Build history of the part. All positions in model axes, mm. A direction names the side the tool comes from. Round coordinates to 2 decimals unless told otherwise and drop trailing zeros. Write each loop counter-clockwise with the first axis right and the second up, starting at its lowest first coordinate (ties: lowest second). Pieces come first, ordered by that corner, then holes.
1) Saw through at B-B (z = 2). Write the cut outline in (x, y).
2) Saw through at C-C (x = 40). Write the cut outline in (y, z).
3) Saw through at A-A (y = 3.8). State how many separate pieces and enclosed holes the cut face has, plus the area to 3 significant figures.
4) Pull direction Z, two halves, no side cores. Call faces 1 (the cylindrical face through (-79.14, 1.01, 17.1)), 2 (the flat face through (-1, 3, -14)), 3 (the cylindrical face through (-79.14, 1.01, -17.1)): +Z half, -Z half, draft (parallel to the pull), parting line (faces both ways), or undercut.
5) Flat gauge pins, fed straight in: pin 1 (2.5 mm diameter, centred on y = 4, z = 2.5, fed in from +X); pin 2 (12 mm diameter, centred on x = 12, z = -5.5, fed in from +Y); pin 3 (2.5 mm diameter, centred on x = -25, y = 3.5, fed in from -Z); pin 4 (2.5 mm diameter, centred on x = 75, z = 13, fed in from -Y). Where does each tip first touch, or does it go through?
6) Saw through at D-D (x = 70). Write the cut outline in (y, z).
7) Wall check: probe 1 along Z at (x, y) = (75, 1.8); probe 2 along X at (y, z) = (1.85, 13); probe 3 along Z at (x, y) = (14, 3.05). Give the ranges that are in metal, low to high.
8) Which spindle directions (+Z, -Z, +X, -X, +Y, -Y) get a long thin tool onto all of the face, cutting with end or side? Do faces 4 (the flat face through (-1, 2, 0)), 5 (the flat face through (-1, 3, -16)), 6 (the flat face through (78, 3, 0)), 7 (the flat face through (-76, 3, 0)). Say none if no direction does.
from build123d import *

# Parameters (mm, degrees)
SKETCH1_W                    = 160
SKETCH1_H                    = 36
BOSS_EXTRUDE1_DEPTH          = 2
SKETCH2_W                    = 130
SKETCH2_H                    = 2
SKETCH2_W_2                  = 2
SKETCH2_H_2                  = 16
BOSS_EXTRUDE2_DEPTH          = 3
CSK_FOR_M3_SFHCS1_AT_2_COUNT = 2
CSK_FOR_M3_SFHCS1_AT_2_PITCH = 26
CIRPATTERN1_COUNT            = 2
FILLET1_R                    = 3
FILLET2_R                    = 1


with BuildPart() as part:
    # Sketch1 → Boss-Extrude1 (new body)
    with BuildSketch(Plane(origin=(0, 0, 0), x_dir=(1, 0, 0), z_dir=(0, 1, 0))):
        Rectangle(SKETCH1_W, SKETCH1_H)
    extrude(amount=BOSS_EXTRUDE1_DEPTH)

    # Sketch2 → Boss-Extrude2 (add)
    with BuildSketch(Plane(origin=(0, 2, 0), x_dir=(1, 0, 0), z_dir=(0, 1, 0))):
        with Locations((0, 15)):
            Rectangle(SKETCH2_W, SKETCH2_H)
        with Locations((77, 0)):
            Rectangle(SKETCH2_W_2, SKETCH2_H_2)
    boss_extrude2 = extrude(amount=BOSS_EXTRUDE2_DEPTH)

    # Sketch7 → CSK for M3 SFHCS1 (revolve, cut)
    with BuildSketch(Plane(origin=(75, 0, -13), x_dir=(0, 0, -1), z_dir=(1, 0, 0))):
        Polygon((0, 0), (0, 11.021463052), (1.7, 10), (1.7, 1.66), (3.36, 0), align=None)
    csk_for_m3_sfhcs1 = revolve(axis=Axis((75, -6.35, -13), (0, 1, 0)), mode=Mode.SUBTRACT)

    # CSK for M3 SFHCS1 at 2: CSK for M3 SFHCS1 ×2
    with Locations(*[(0, 0, i * CSK_FOR_M3_SFHCS1_AT_2_PITCH) for i in range(1, CSK_FOR_M3_SFHCS1_AT_2_COUNT)]):
        add(csk_for_m3_sfhcs1, mode=Mode.SUBTRACT)

    # CirPattern1: Boss-Extrude2, CSK for M3 SFHCS1 ×2 about axis
    cirpattern1_axis = Axis((0, 0, 0), (0, 1, 0))
    add([boss_extrude2.rotate(cirpattern1_axis, i * 360 / CIRPATTERN1_COUNT) for i in range(1, CIRPATTERN1_COUNT)])
    add([csk_for_m3_sfhcs1.rotate(cirpattern1_axis, i * 360 / CIRPATTERN1_COUNT) for i in range(1, CIRPATTERN1_COUNT)], mode=Mode.SUBTRACT)

    # CirPattern1 copy 1 sketch → CirPattern1 copy 1 (revolve, cut)
    with BuildSketch(Plane(origin=(-75, 0, -13), x_dir=(0, 0, 1), z_dir=(-1, 0, 0))):
        Polygon((0, 0), (0, 11.021463052), (1.7, 10), (1.7, 1.66), (3.36, 0), align=None)
    revolve(axis=Axis((-75, -6.35, -13), (0, 1, 0)), mode=Mode.SUBTRACT)

    # Fillet1
    fillet1_edges = [part.edges().sort_by_distance(p)[0] for p in [
        (-80, 1, -18),
        (80, 1, -18),
        (80, 1, 18),
        (-80, 1, 18),
    ]]
    fillet(fillet1_edges, radius=FILLET1_R)

    # Fillet2
    fillet2_edges = [part.edges().sort_by_distance(p)[0] for p in [
        (-78, 3.5, -8),
        (-78, 3.5, 8),
        (-76, 3.5, 8),
        (-76, 3.5, -8),
        (-65, 3.5, 14),
        (-65, 3.5, 16),
        (65, 3.5, 16),
        (65, 3.5, 14),
        (78, 3.5, 8),
        (78, 3.5, -8),
        (76, 3.5, -8),
        (76, 3.5, 8),
        (65, 3.5, -14),
        (65, 3.5, -16),
        (-65, 3.5, -16),
        (-65, 3.5, -14),
    ]]
    fillet(fillet2_edges, radius=FILLET2_R - 0.0001)  # a hair under: the kernel refuses the full size


solid = part.part
Evaluation:
1. outline: (-80, 0) - (80, 0) - (80, 2) - (78, 2) - (78, 5) - (76, 5) - (76, 2) - (-76, 2) - (-76, 5) - (-78, 5) - (-78, 2) - (-80, 2) - close
2. outline: (0, -18) - (2, -18) - (2, -16) - (5, -16) - (5, -14) - (2, -14) - (2, 14) - (5, 14) - (5, 16) - (2, 16) - (2, 18) - (0, 18) - close
3. separate pieces: 4
3. enclosed holes: 0
3. area: 581 mm2
4. face 1: +Z half
4. face 2: undercut
4. face 3: -Z half
5. pin 1: stops at x = 78
5. pin 2: stops at y = 2
5. pin 3: stops at z = -16
5. pin 4: passes through
6. outline: (0, -18) - (2, -18) - (2, 18) - (0, 18) - close
7. probe 1: z = -18 to -14.7, -11.3 to 11.3, 14.7 to 18
7. probe 2: x = -80 to -76.7, -73.3 to 73.3, 76.7 to 80
7. probe 3: z = -16 to -14, 14 to 16
8. face 4: +Y
8. face 5: -Z, +X, -X, +Y
8. face 6: +Z, -Z, +X, +Y
8. face 7: +Z, -Z, +Y
